CAD build for the part. Positions are in the model's coordinates, mm. A direction names the side the tool comes from. Coordinates: 2 decimals unless noted, no trailing zeros. Loops run counter-clockwise (first coordinate to the right, second up) from the corner with the lowest first, then second, coordinate; pieces in that order, holes last. Notation, with made-up numbers: (-15, 4.25) -> (24, 4.25) arc R20 ccw to (24, 39.25) -> close; hole circle Ø11 at (63, 37). An arc over 180 degrees is marked (long way). Write each question's results on one line, items separated by ' | '.
from build123d import *

# Parameters (mm, degrees)
P_IDAT_VYSUNUT_M1_DEPTH  = 4
SKICA2_W                 = 5
SKICA2_H                 = 8
P_IDAT_VYSUNUT_M2_DEPTH  = 20
SKICA3_W                 = 8
SKICA3_H                 = 5
P_IDAT_VYSUNUT_M3_DEPTH  = 32
SKICA5_R                 = 2.04
ODEBRAT_VYSUNUT_M1_DEPTH = 15
ZAOBLIT1_R               = 5
SKICA6_R                 = 1.2
ODEBRAT_VYSUNUT_M2_DEPTH = 8
ZAOBLIT2_R               = 4
SKICA7_R                 = 0.95
ODEBRAT_VYSUNUT_M3_DEPTH = 13
SCALE1_SCALE             = 8


with BuildPart() as part:
    # Skica1 → Přidat vysunutím1 (new, symmetric)
    with BuildSketch(Plane.XY):
        Polygon((0, 0), (17, 0), (17, 23.5), (0, 23.5), (0, 28.5), (22, 28.5), (22, -5), (0, -5), align=None)
    extrude(amount=P_IDAT_VYSUNUT_M1_DEPTH, both=True)

    # Skica2 → Přidat vysunutím2 (add)
    with BuildSketch(Plane(origin=(0, 28.5, 0), x_dir=(1, 0, 0), z_dir=(0, 1, 0))):
        with Locations((19.5, 0)):
            Rectangle(SKICA2_W, SKICA2_H)
    extrude(amount=P_IDAT_VYSUNUT_M2_DEPTH)

    # Skica3 → Přidat vysunutím3 (add)
    with BuildSketch(Plane.ZY.offset(-17)):
        with Locations((0, 46)):
            Rectangle(SKICA3_W, SKICA3_H)
    extrude(amount=P_IDAT_VYSUNUT_M3_DEPTH)

    # Skica5 → Odebrat vysunutím1 (cut)
    with BuildSketch(Plane(origin=(0, 48.5, 0), x_dir=(1, 0, 0), z_dir=(0, 1, 0))):
        with Locations(Location((-2, 0, 0), (0, 0, 270))):
            Circle(SKICA5_R)
    extrude(amount=-ODEBRAT_VYSUNUT_M1_DEPTH, mode=Mode.SUBTRACT)

    # Zaoblit1
    zaoblit1_edges = [part.edges().sort_by_distance(p)[0] for p in [
        (22, -5, 0),
        (22, 48.5, 0),
    ]]
    fillet(zaoblit1_edges, radius=ZAOBLIT1_R)

    # Skica6 → Odebrat vysunutím2 (cut)
    with BuildSketch(Plane.ZY):
        with Locations((-6.1415e-05, 25.09368658)):
            Circle(SKICA6_R)
        with Locations((-5.8558e-05, -1.893787552)):
            Circle(SKICA6_R)
    extrude(amount=-ODEBRAT_VYSUNUT_M2_DEPTH, mode=Mode.SUBTRACT)

    # Zaoblit2
    zaoblit2_edges = [part.edges().sort_by_distance(p)[0] for p in [
        (-15, 46, -4),
        (-15, 46, 4),
    ]]
    fillet(zaoblit2_edges, radius=ZAOBLIT2_R - 0.0001)  # a hair under: the kernel refuses the full size

    # Skica7 → Odebrat vysunutím3 (cut)
    with BuildSketch(Plane(origin=(0, 48.5, 0), x_dir=(1, 0, 0), z_dir=(0, 1, 0))):
        with Locations(Location((-10.5, 0, 0), (0, 0, 270))):
            Circle(SKICA7_R)
        with Locations(Location((6.5, 0, 0), (0, 0, 270))):
            Circle(SKICA7_R)
    extrude(amount=-ODEBRAT_VYSUNUT_M3_DEPTH, mode=Mode.SUBTRACT)


with BuildPart() as part_1:
    # Scale1: scaled about (11.829762973, 25.103410302, 9.66e-07)
    add(part.part.scale(SCALE1_SCALE).moved(Location((-82.808340811, -175.723872114, -6.762e-06))))


solid = part_1.part
1) Drill centre lines: L1, parallel to Y at x = 46.5, z = 17.5; L2, parallel to Z at x = -167, y = 173.5; L3, parallel to X at y = 60, z = 23.5. Where is each one in solid material? Low to high. Write a range as from..to.
Outcome:
L1: y = -215.72..-175.72, 12.28..52.28, 172.28..212.28 | L2: z = -32..-7.6, 7.6..32 | L3: x = 53.19..93.19
2) Slice it at D-D (y = 122). Write the cut outline in (x, z).
Outcome:
outline: (53.19, -32) -> (93.19, -32) -> (93.19, 32) -> (53.19, 32) -> close
3) Two-plate mould, pull along X, no slides. Class faces 1 (the cylindrical face through (-37.55, 192.56, 3.51)), 2 (the flat face through (-73, 172.276, 0)), 3 (the cylindrical face through (-193.68, 192.56, 22.38)): pulls with the +X half, pulls with the -X half, needs draft (parallel to the pull), parting line crosses it, or undercut.
Outcome:
face 1: undercut | face 2: needs draft | face 3: pulls with the -X half
4) Slice it at C-C (z = -27). Write the cut outline in (x, y).
Outcome:
outline: (-187.98, 172.28) -> (53.19, 172.28) -> (53.19, 52.28) -> (-82.81, 52.28) -> (-82.81, 12.28) -> (53.19, 12.28) -> (53.19, -175.72) -> (-82.81, -175.72) -> (-82.81, -215.72) -> (53.19, -215.72) arc R40 ccw to (93.19, -175.72) -> (93.19, 172.28) arc R40 ccw to (53.19, 212.28) -> (-187.98, 212.28) -> close
5) Pin check, flat tips, straight feed: pin 1 (12 mm diameter, centred on y = 165.5, z = 4.5, fed in from -X); pin 2 (21 mm diameter, centred on y = -191.5, z = 2.5, fed in from -X); pin 3 (1 mm diameter, centred on x = 55, z = 21, fed in from -Y). Stop position of each tip, or through.
Outcome:
pin 1: stops at x = 53.19 | pin 2: stops at x = -82.81 | pin 3: stops at y = -215.7
6) Slice it at A-A (x = -13.5). Write the cut outline in (y, z).
Outcome:
outline: (-215.72, -32) -> (-175.72, -32) -> (-175.72, 32) -> (-215.72, 32) -> close; (12.28, -32) -> (52.28, -32) -> (52.28, 32) -> (12.28, 32) -> close; (172.28, -32) -> (212.28, -32) -> (212.28, 32) -> (172.28, 32) -> close
7) Slice it at B-B (y = 184.5). Count the separate pieces of the cut face and the enclosed holes in it, then the cut area to 3 significant figures.
Outcome:
separate pieces: 1 | enclosed holes: 3 | area: 17,200 mm^2
8) Which spindle directions (+Z, -Z, +X, -X, +Y, -Y) get a long thin tool onto all of the face, cutting with end or side? Do faces 4 (the flat face through (-82.808, -200, 8)), 5 (the flat face through (-16, -175.724, 0)), 6 (the cylindrical face through (-51.256, -181.356, -1.25)). Say none if no direction does.
Outcome:
face 4: +Z, -Z, -X, -Y | face 5: +Z, -Z, -X | face 6: -X
